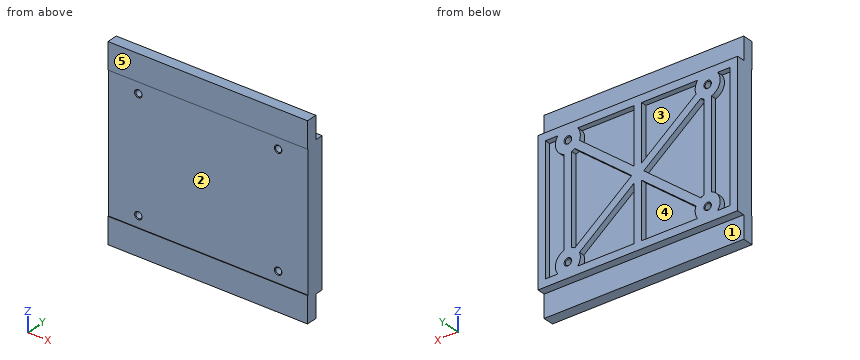
from build123d import *

# Parameters (mm, degrees)
BOSS_EXTRUDE1_DEPTH = 80
SKETCH2_W           = 80
SKETCH2_H           = 57
BOSS_EXTRUDE2_DEPTH = 2.25


with BuildPart() as part:
    # Sketch1 → Boss-Extrude1 (new body)
    with BuildSketch(Plane(origin=(0, 0, 0), x_dir=(0, 0, -1), z_dir=(1, 0, 0))):
        Polygon((-37.5, 4.5), (-27, 4.5), (-27, 4.75), (27, 4.75), (27, 4.5), (37.5, 4.5), (37.5, 8.8), (28.5, 8.8), (28.5, 9.75), (-28.5, 9.75), (-28.5, 8.8), (-37.5, 8.8), align=None)
    extrude(amount=BOSS_EXTRUDE1_DEPTH)

    # Sketch2 → Boss-Extrude2 (add)
    with BuildSketch(Plane(origin=(0, 9.75, 0), x_dir=(1, 0, 0), z_dir=(0, 1, 0))):
        with Locations((40, 0)):
            Rectangle(SKETCH2_W, SKETCH2_H)
        with BuildLine():
            Line((69.5, 17.730303993), (69.5, -17.730303993))
            ThreePointArc((69.5, -17.730303993), (72.759678982, -20.968511838), (72, -25.5))
            Line((72, -25.5), (77, -25.5))
            Line((77, -25.5), (77, 25.5))
            Line((77, 25.5), (72, 25.5))
            ThreePointArc((72, 25.5), (72.759678982, 20.968511838), (69.5, 17.730303993))
        make_face(mode=Mode.SUBTRACT)
        with BuildLine():
            Line((42.394670007, 0), (65.221566009, -18.34304143))
            ThreePointArc((65.221566009, -18.34304143), (65.838956006, -17.991132198), (66.5, -17.730303993))
            Line((66.5, -17.730303993), (66.5, 17.730303993))
            ThreePointArc((66.5, 17.730303993), (65.838956006, 17.991132198), (65.221566009, 18.34304143))
            Line((65.221566009, 18.34304143), (42.394670007, 0))
        make_face(mode=Mode.SUBTRACT)
        with BuildLine():
            Line((41.5, 25.5), (41.5, 3.129645542))
            Line((41.5, 3.129645542), (63.342392684, 20.681568234))
            ThreePointArc((63.342392684, 20.681568234), (63.045924679, 23.176119604), (64, 25.5))
            Line((64, 25.5), (41.5, 25.5))
        make_face(mode=Mode.SUBTRACT)
        with BuildLine():
            Line((41.5, -25.5), (64, -25.5))
            ThreePointArc((64, -25.5), (63.045924679, -23.176119604), (63.342392684, -20.681568234))
            Line((63.342392684, -20.681568234), (41.5, -3.129645542))
            Line((41.5, -3.129645542), (41.5, -25.5))
        make_face(mode=Mode.SUBTRACT)
        with BuildLine():
            Line((16.657607316, 20.681568234), (38.5, 3.129645542))
            Line((38.5, 3.129645542), (38.5, 25.5))
            Line((38.5, 25.5), (16, 25.5))
            ThreePointArc((16, 25.5), (16.954075321, 23.176119604), (16.657607316, 20.681568234))
        make_face(mode=Mode.SUBTRACT)
        with BuildLine():
            Line((16, -25.5), (38.5, -25.5))
            Line((38.5, -25.5), (38.5, -3.129645542))
            Line((38.5, -3.129645542), (16.657607316, -20.681568234))
            ThreePointArc((16.657607316, -20.681568234), (16.954075321, -23.176119604), (16, -25.5))
        make_face(mode=Mode.SUBTRACT)
        with BuildLine():
            Line((14.778433991, -18.34304143), (37.605329993, 0))
            Line((37.605329993, 0), (14.778433991, 18.34304143))
            ThreePointArc((14.778433991, 18.34304143), (14.161043994, 17.991132198), (13.5, 17.730303993))
            Line((13.5, 17.730303993), (13.5, -17.730303993))
            ThreePointArc((13.5, -17.730303993), (14.161043994, -17.991132198), (14.778433991, -18.34304143))
        make_face(mode=Mode.SUBTRACT)
        with BuildLine():
            Line((3, -25.5), (8, -25.5))
            ThreePointArc((8, -25.5), (7.240321018, -20.968511838), (10.5, -17.730303993))
            Line((10.5, -17.730303993), (10.5, 17.730303993))
            ThreePointArc((10.5, 17.730303993), (7.240321018, 20.968511838), (8, 25.5))
            Line((8, 25.5), (3, 25.5))
            Line((3, 25.5), (3, -25.5))
        make_face(mode=Mode.SUBTRACT)
    extrude(amount=BOSS_EXTRUDE2_DEPTH)

    # Sketch3 → Cut-Revolve1 (revolve, cut)
    with BuildSketch(Plane.XY.offset(22.5), mode=Mode.PRIVATE) as cut_revolve1_sk:
        Polygon((12, 12), (13.5, 12), (13.2295, 11.7295), (13.2295, 5.0205), (13.5, 4.75), (12, 4.75), align=None)
    revolve(cut_revolve1_sk.sketch.rotate(Axis((12, 4.75, 22.5), (0, 1, 0)), 270), axis=Axis((12, 4.75, 22.5), (0, 1, 0)), mode=Mode.SUBTRACT)

    # Sketch4 → Cut-Revolve2 (revolve, cut)
    with BuildSketch(Plane.XY.offset(22.5), mode=Mode.PRIVATE) as cut_revolve2_sk:
        Polygon((68, 12), (69.5, 12), (69.2295, 11.7295), (69.2295, 5.0205), (69.5, 4.75), (68, 4.75), align=None)
    revolve(cut_revolve2_sk.sketch.rotate(Axis((68, 4.75, 22.5), (0, 1, 0)), 270), axis=Axis((68, 4.75, 22.5), (0, 1, 0)), mode=Mode.SUBTRACT)

    # Sketch5 → Cut-Revolve3 (revolve, cut)
    with BuildSketch(Plane.XY.offset(-22.5), mode=Mode.PRIVATE) as cut_revolve3_sk:
        Polygon((12, 12), (13.5, 12), (13.2295, 11.7295), (13.2295, 5.0205), (13.5, 4.75), (12, 4.75), align=None)
    revolve(cut_revolve3_sk.sketch.rotate(Axis((12, 4.75, -22.5), (0, 1, 0)), 270), axis=Axis((12, 4.75, -22.5), (0, 1, 0)), mode=Mode.SUBTRACT)

    # Sketch6 → Cut-Revolve4 (revolve, cut)
    with BuildSketch(Plane.XY.offset(-22.5), mode=Mode.PRIVATE) as cut_revolve4_sk:
        Polygon((68, 12), (69.5, 12), (69.2295, 11.7295), (69.2295, 5.0205), (69.5, 4.75), (68, 4.75), align=None)
    revolve(cut_revolve4_sk.sketch.rotate(Axis((68, 4.75, -22.5), (0, 1, 0)), 270), axis=Axis((68, 4.75, -22.5), (0, 1, 0)), mode=Mode.SUBTRACT)


solid = part.part
Model file for the job. Use its own axes, mm. Face numbers are marked on the shaded views. A direction names the side the tool comes from. Give positions to 0.01 mm unless a question says otherwise; leave off trailing zeros. Order: outer loops, then holes, each group sorted by start corner. A loop starts at its lowest first (then second) coordinate and runs counter-clockwise, first axis right, second up. Notation, with made-up numbers: M 6.25,-3.5 L 22.25,-3.5 A10 ccw 22.25,2.5 Z; hole C 57,-24 d10. An arc over 180 degrees is marked long. Put each result on its own line as item: value. Start each with the question number.
(1) Pin check, flat tips, straight feed: pin 1 Ø6.5 at (x, z) = (29, 16.5) entering from +Y; pin 2 Ø1.5 at (x, z) = (68, -22.5) entering from -Y; pin 3 Ø2.5 at (x, y) = (30, 11) entering from +Z; pin 4 Ø3.5 at (x, y) = (25.5, 11) entering from -Z. Stop position of each tip, or through.
(2) Pull direction X, two halves, no side cores. Call the marked faces 4 and 5: released by +X, released by -X, zero draft, split by the parting line, or undercut.
(3) Tool access for the marked faces 1, 2 and 3: list every direction of +Z, -Z, +X, -X, +Y, -Y with a clear straight run to the whole face (end or side of a thin tool).
(4) Band-saw the part on A-A on x = 68. Give the cut face in (y, z).
(5) Band-saw the part on D-D on x = 25. Give the cut face in (y, z), then the cut area to 3 significant figures.
(6) Band-saw the part on C-C on z = -22.5. Count the separate pieces of the cut face and the enclosed holes in it, then the cut area to 3 significant figures.
(7) Band-saw the part on B-B on z = 10. Give the cut face in (x, y).
(8) Drill centre lines: L1, parallel to X at y = 7.75, z = 22.5; L2, parallel to Z at x = 68, y = 9.5; L3, parallel to Z at x = 6.5, y = 10.5. Where is each one in solid material? Low to high. Write a range as [from, to].
Results below:
1. pin 1: stops at y = 9.75
1. pin 2: passes through
1. pin 3: stops at z = 28.5
1. pin 4: stops at z = -28.5
2. face 4: undercut
2. face 5: zero draft
3. face 1: -Z, +X, -X, +Y
3. face 2: +X, -X, -Y
3. face 3: +Y
4. outline: M 4.5,-37.5 L 8.8,-37.5 L 8.8,-28.5 L 12,-28.5 L 12,-24 L 11.73,-23.73 L 5.02,-23.73 L 4.75,-24 L 4.75,-27 L 4.5,-27 Z; M 4.5,27 L 4.75,27 L 4.75,24 L 5.02,23.73 L 11.73,23.73 L 12,24 L 12,28.5 L 8.8,28.5 L 8.8,37.5 L 4.5,37.5 Z; M 4.75,-21 L 5.02,-21.27 L 11.73,-21.27 L 12,-21 L 12,21 L 11.73,21.27 L 5.02,21.27 L 4.75,21 Z
5. outline: M 4.5,-37.5 L 8.8,-37.5 L 8.8,-28.5 L 12,-28.5 L 12,-25.5 L 9.75,-25.5 L 9.75,-13.98 L 12,-13.98 L 12,-10.13 L 9.75,-10.13 L 9.75,10.13 L 12,10.13 L 12,13.98 L 9.75,13.98 L 9.75,25.5 L 12,25.5 L 12,28.5 L 8.8,28.5 L 8.8,37.5 L 4.5,37.5 L 4.5,27 L 4.75,27 L 4.75,-27 L 4.5,-27 Z
5. area: 394 mm2
6. separate pieces: 3
6. enclosed holes: 0
6. area: 429 mm2
7. outline: M 0,4.75 L 80,4.75 L 80,12 L 77,12 L 77,9.75 L 69.5,9.75 L 69.5,12 L 66.5,12 L 66.5,9.75 L 54.84,9.75 L 54.84,12 L 50.05,12 L 50.05,9.75 L 41.5,9.75 L 41.5,12 L 38.5,12 L 38.5,9.75 L 29.95,9.75 L 29.95,12 L 25.16,12 L 25.16,9.75 L 13.5,9.75 L 13.5,12 L 10.5,12 L 10.5,9.75 L 3,9.75 L 3,12 L 0,12 Z
8. L1: x = [0, 10.77], [13.23, 66.77], [69.23, 80]
8. L2: z = [-28.5, -23.73], [-21.27, 21.27], [23.73, 28.5]
8. L3: z = [-28.5, -25.5], [25.5, 28.5]
